from build123d import *

# Parameters (mm, degrees)
BOSS_EXTRUDE1_DEPTH = 5


with BuildPart() as part:
    # Sketch1 → Boss-Extrude1 (new, symmetric)
    with BuildSketch(Plane.XY):
        with BuildLine():
            Line((-47, 51), (47, 51))
            ThreePointArc((47, 51), (49.828427125, 49.828427125), (51, 47))
            Line((51, 47), (51, -47))
            ThreePointArc((51, -47), (49.828427125, -49.828427125), (47, -51))
            Line((47, -51), (-47, -51))
            ThreePointArc((-47, -51), (-49.828427125, -49.828427125), (-51, -47))
            Line((-51, -47), (-51, 47))
            ThreePointArc((-51, 47), (-49.828427125, 49.828427125), (-47, 51))
        make_face()
        with BuildLine():
            Line((-18.935786438, 24.335135157), (-18.935786438, 24.5))
            ThreePointArc((-18.935786438, 24.5), (-18.239751149, 26.963133018), (-16.192917188, 28.5))
            Line((-16.192917188, 28.5), (16.192917188, 28.5))
            ThreePointArc((16.192917188, 28.5), (18.239751149, 26.963133018), (18.935786438, 24.5))
            Line((18.935786438, 24.5), (18.935786438, 24.335135157))
            ThreePointArc((18.935786438, 24.335135157), (20.272310951, 20.112043563), (24.314285714, 18.300072152))
            Line((24.314285714, 18.300072152), (25.314285714, 18.300072152))
            ThreePointArc((25.314285714, 18.300072152), (27.253927817, 17.467886008), (28.5, 15.76434576))
            Line((28.5, 15.76434576), (28.5, -16.192917188))
            ThreePointArc((28.5, -16.192917188), (26.963133018, -18.239751149), (24.5, -18.935786438))
            Line((24.5, -18.935786438), (24.335135157, -18.935786438))
            ThreePointArc((24.335135157, -18.935786438), (20.112043563, -20.272310951), (18.300072152, -24.314285714))
            Line((18.300072152, -24.314285714), (18.300072152, -25.314285714))
            ThreePointArc((18.300072152, -25.314285714), (17.467886008, -27.253927817), (15.76434576, -28.5))
            Line((15.76434576, -28.5), (-15.76434576, -28.5))
            ThreePointArc((-15.76434576, -28.5), (-17.467886008, -27.253927817), (-18.300072152, -25.314285714))
            Line((-18.300072152, -25.314285714), (-18.300072152, -24.314285714))
            ThreePointArc((-18.300072152, -24.314285714), (-20.112043563, -20.272310951), (-24.335135157, -18.935786438))
            Line((-24.335135157, -18.935786438), (-24.5, -18.935786438))
            ThreePointArc((-24.5, -18.935786438), (-26.963133018, -18.239751149), (-28.5, -16.192917188))
            Line((-28.5, -16.192917188), (-28.5, 15.76434576))
            ThreePointArc((-28.5, 15.76434576), (-27.253927817, 17.467886008), (-25.314285714, 18.300072152))
            Line((-25.314285714, 18.300072152), (-24.314285714, 18.300072152))
            ThreePointArc((-24.314285714, 18.300072152), (-20.272310951, 20.112043563), (-18.935786438, 24.335135157))
        make_face(mode=Mode.SUBTRACT)
    extrude(amount=BOSS_EXTRUDE1_DEPTH, both=True)


solid = part.part
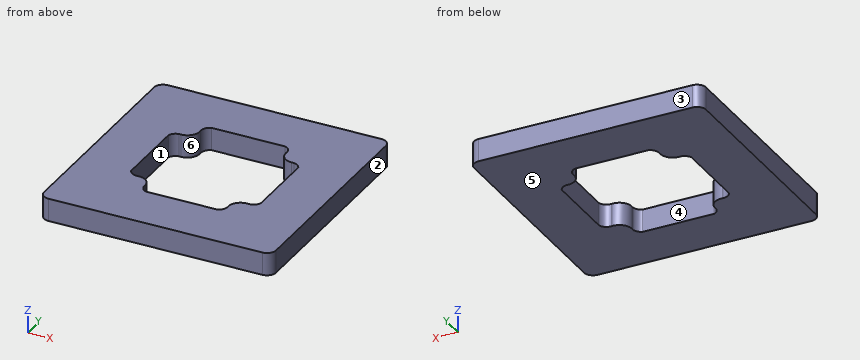
The model under review builds one solid part; all positions refer to its coordinate system, in mm. Face numbers are marked on the shaded views. A direction names the side the tool comes from. Give positions to 0.01 mm unless a question says otherwise; leave off trailing zeros. Order: outer loops, then holes, each group sorted by start corner. A loop starts at its lowest first (then second) coordinate and runs counter-clockwise, first axis right, second up. Notation, with made-up numbers: (-11.75, 62.5) -> (18.25, 62.5) arc R34 ccw to (18.25, 101.5) -> close; hole circle Ø10 at (88, -26). An arc over 180 degrees is marked (long way). Write item = value, one per line. Start each with the question number.
(1) Take a section at B-B (x = -14). Write out the cut boundary in (y, z).
(2) For L1, parallel to X at y = -12, z = -2.5; L2, parallel to X at y = 24.5, z = 0, list the stretches that pass through material, from the lowest coordinate up. Write a range as from..to.
(3) Draft analysis for pull direction Y (two halves, no side actions). For the marked faces 1, 2, 3 and 4, state which applies: +Y half, -Y half, draft (parallel to the pull), parting line (faces both ways), or undercut.
(4) Tool access review of the marked faces 5 and 6: name each direction out of +Z, -Z, +X, -X, +Y, -Y from which nothing blocks a thin tool from reaching the whole face with its end or side.
Returned:
q1.outline = (-51, -5) -> (-28.5, -5) -> (-28.5, 5) -> (-51, 5) -> close; (28.5, -5) -> (51, -5) -> (51, 5) -> (28.5, 5) -> close
q2.L1 = -51..-28.5, 28.5..51
q2.L2 = -51..-18.94, 18.94..51
q3.face_1 = undercut
q3.face_2 = draft
q3.face_3 = +Y half
q3.face_4 = undercut
q4.face_5 = -Z, +X, -X, +Y, -Y
q4.face_6 = +Z, -Z
